The drawing under review shows one solid part. Ordinate dimensions are in mm from its lowest x, y, z. A direction names the side the tool comes from. Coordinates: 2 decimals unless noted, no trailing zeros. Loops run counter-clockwise (first coordinate to the right, second up) from the corner with the lowest first, then second, coordinate; pieces in that order, holes last. Notation, with made-up numbers: M -33,53 L -8,53 A17 ccw -8,77 Z; hole C -11,31 d3. An arc over 180 degrees is marked long. Put each result on its own line as item: value.
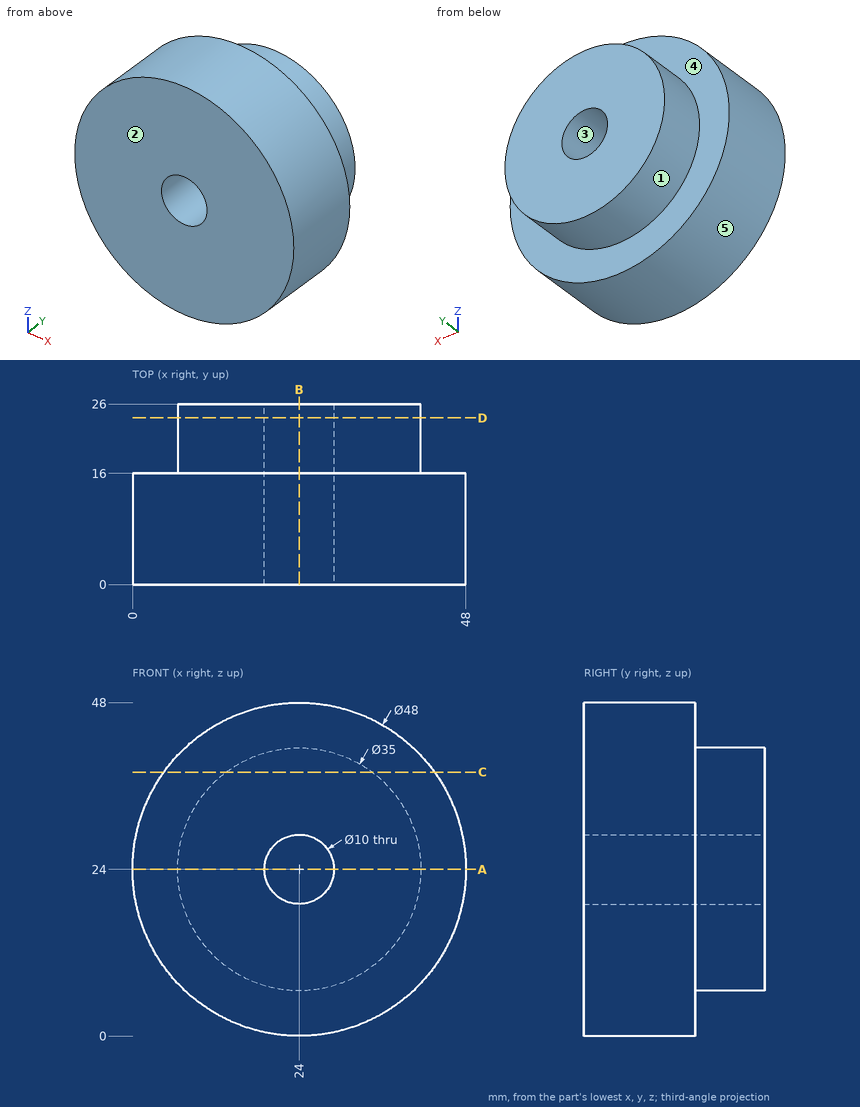
(1) Add section B-B (x = 24). Write out the cut boundary in (y, z).
Determined:
outline: M 0,0 L 16,0 L 16,6.5 L 26,6.5 L 26,19 L 0,19 Z; M 0,29 L 26,29 L 26,41.5 L 16,41.5 L 16,48 L 0,48 Z
(2) Add section D-D (y = 24). Write out the cut boundary in (x, z), plus the area to 3 significant figures.
Determined:
outline: C 24,24 d35; hole C 24,24 d10
area: 884 mm^2
(3) For pin 1 (8 mm diameter, centred on x = 25, y = 14.5, fed in from +Z); pin 2 (2 mm diameter, centred on x = 42, y = 13.5, fed in from -Z); pin 3 (10 mm diameter, centred on x = 10.5, y = 10.5, fed in from +Z), all flat-tipped, find the tip position at first contact; note any pin that passes through.
Determined:
pin 1: stops at z = 48
pin 2: stops at z = 7.06
pin 3: stops at z = 46.44
(4) Wall thickness on line 1 along Z through (x, y) = (24, 15); line 2 along Z through (x, y) = (24, 20): over which ranges is each line inside the solid? List them lowest first. Write a range as [from, to].
Determined:
line 1: z = [0, 19], [29, 48]
line 2: z = [6.5, 19], [29, 41.5]
(5) Add section A-A (z = 24). Write out the cut boundary in (x, y), plus the area to 3 significant figures.
Determined:
outline: M 0,0 L 19,0 L 19,26 L 6.5,26 L 6.5,16 L 0,16 Z; M 29,0 L 48,0 L 48,16 L 41.5,16 L 41.5,26 L 29,26 Z
area: 858 mm^2
(6) Tool access review of the marked faces 1 and 2: name each direction out of +Z, -Z, +X, -X, +Y, -Y from which nothing blocks a thin tool from reaching the whole face with its end or side.
Determined:
face 1: +Y
face 2: +Z, -Z, +X, -X, -Y
(7) Draft analysis for pull direction X (two halves, no side actions). For the marked faces 3, 4 and 5, state which applies: +X half, -X half, draft (parallel to the pull), parting line (faces both ways), or undercut.
Determined:
face 3: undercut
face 4: draft
face 5: parting line
(8) Add section C-C (z = 38). Write out the cut boundary in (x, y).
Determined:
outline: M 4.51,0 L 43.49,0 L 43.49,16 L 34.5,16 L 34.5,26 L 13.5,26 L 13.5,16 L 4.51,16 Z
